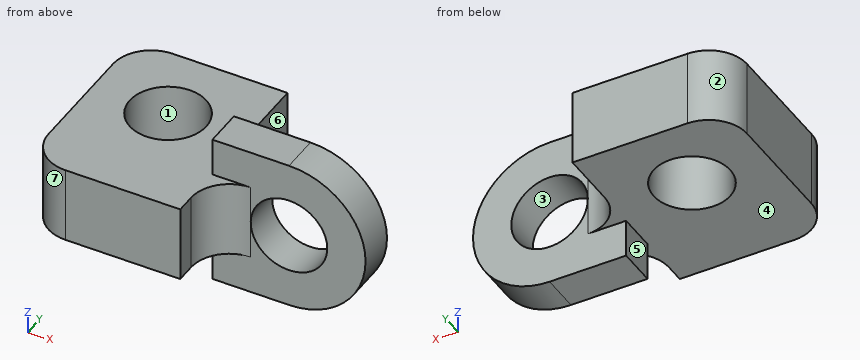
```python
from build123d import *

# Parameters (mm, degrees)
SKETCH_1_R      = 5
EXTRUDE_1_DEPTH = 2.5
SKETCH_2_R      = 5
EXTRUDE_2_DEPTH = 5
FILLET_1_R      = 5


with BuildPart() as part:
    # 草圖1 → 填料-伸長1 (new, symmetric)
    with BuildSketch(Plane(origin=(0, 0, 0), x_dir=(1, 0, 0), z_dir=(0, 1, 0))):
        with BuildLine():
            Line((0, 10), (-10, 10))
            Line((-10, 10), (-10, -10))
            Line((-10, -10), (0, -10))
            ThreePointArc((0, -10), (10, 0), (0, 10))
        make_face()
        with Locations(Location((0, 0, 0), (0, 0, 270))):
            Circle(SKETCH_1_R, mode=Mode.SUBTRACT)
    extrude(amount=EXTRUDE_1_DEPTH, both=True)

    # 草圖2 → 填料-伸長2 (add, symmetric)
    with BuildSketch(Plane.XY):
        with BuildLine():
            Line((-30, 1.898257061), (-30, -5))
            ThreePointArc((-30, -5), (-28.535533906, -8.535533906), (-25, -10))
            Line((-25, -10), (-10, -10))
            Line((-10, -10), (-10, -2.5))
            Line((-10, -2.5), (-10, 2.5))
            Line((-10, 2.5), (-10, 15))
            Line((-10, 15), (-25, 15))
            ThreePointArc((-25, 15), (-28.535533906, 13.535533906), (-30, 10))
            Line((-30, 10), (-30, 1.898257061))
        make_face()
        with Locations((-20, 5)):
            Circle(SKETCH_2_R, mode=Mode.SUBTRACT)
    extrude(amount=EXTRUDE_2_DEPTH, both=True)

    # 圓角1
    fillet_1_edges = [part.edges().sort_by_distance(p)[0] for p in [
        (-10, -2.5, 0),
        (-10, 2.5, 0),
    ]]
    fillet(fillet_1_edges, radius=FILLET_1_R)


solid = part.part
```
Read the model definition and answer for the solid it produces. Units are mm, in the model's axes. Face numbers are marked on the shaded views. A direction names the side the tool comes from. Round coordinates to 2 decimals unless told otherwise and drop trailing zeros. Write each loop counter-clockwise with the first axis right and the second up, starting at its lowest first coordinate (ties: lowest second). Pieces come first, ordered by that corner, then holes. Notation, with made-up numbers: (-23.75, -35.5) - (-6.75, -35.5) arc R32 cw to (-6.75, 3.5) - close; hole circle Ø9 at (16, -37). An arc over 180 degrees is marked (long way). Use CSV: the item, a comma, the result in double quotes.
Q1. Find section A-A, the plane x = -4. Write down the section's boundary in (y, z).
Values:
outline,"(-2.5, -10) - (2.5, -10) - (2.5, -3) - (-2.5, -3) - close; (-2.5, 3) - (2.5, 3) - (2.5, 10) - (-2.5, 10) - close"
Q2. Straight lines are drawn through the part: line 1 along X through (y, z) = (2, -0.5); line 2 along Z through (x, y) = (-26, -3.25); line 3 along Y through (x, z) = (-22, 0.5). For each, find the intervals that lie inside material, in ascending order.
Values:
line 1,"x = -30 to -24, -16 to -4.97, 4.97 to 9.99"
line 2,"z = -5 to 5"
line 3,"y = -10 to 0.42, 9.58 to 15"
Q3. Find section D-D, the plane z = 2.75. Write down the section's boundary in (x, y), then the cut area to 3 significant figures.
Values:
outline,"(-30, -5) arc R5 ccw to (-25, -10) - (-10, -10) - (-10, -7.5) arc R5 cw to (-5, -2.5) - (-4.18, -2.5) - (-4.18, 2.5) - (-5, 2.5) arc R5 cw to (-10, 7.5) - (-10, 15) - (-25, 15) arc R5 ccw to (-30, 10) - close; (4.18, -2.5) - (9.61, -2.5) - (9.61, 2.5) - (4.18, 2.5) - close; hole circle Ø10 at (-20, 5)"
area,"478 mm²"
Q4. Determine the mould class of the marked faces 1, 2, 3 and 4 for opening direction X: +X half, -X half, draft (parallel to the pull), parting line (faces both ways), or undercut.
Values:
face 1,"undercut"
face 2,"-X half"
face 3,"undercut"
face 4,"draft"
Q5. Each of these flat-tipped pins is pushed along its axis until it touches: pin 1 Ø1.3 at (y, z) = (-9, 1) entering from +X; pin 2 Ø1.5 at (y, z) = (0.5, -6.5) entering from -X; pin 3 Ø9 at (x, z) = (0, 0) entering from -Y; pin 4 Ø2 at (x, y) = (-20, 11.5) entering from -Z. Where does it stop, or does it pass through?
Values:
pin 1,"stops at x = -10"
pin 2,"stops at x = -10"
pin 3,"passes through"
pin 4,"stops at z = -5"
Q6. A tool of negligible diameter and unlimited length cuts with its end or side. For the marked faces 5, 6 and 7, from which of +Z, -Z, +X, -X, +Y, -Y can it reach the whole face along a straight path? Write none if from no direction.
Values:
face 5,"-Z, -X, +Y, -Y"
face 6,"+Z, -Z, +X, +Y"
face 7,"+Z, -Z, -X, -Y"
Q7. Find section B-B, the plane z = 0.25. Count the separate pieces of the cut face and the enclosed holes in it, then the cut area to 3 significant figures.
Values:
separate pieces,"2"
enclosed holes,"1"
area,"472 mm²"
Q8. Find section C-C, the plane y = 5. Write down the section's boundary in (x, z), then the cut area to 3 significant figures.
Values:
outline,"(-30, -5) - (-25, -5) - (-25, 5) - (-30, 5) - close; (-15, -5) - (-9.33, -5) - (-9.33, 5) - (-15, 5) - close"
area,"107 mm²"
